Here's how the part is built. I have some questions about the finished solid (model axes, mm). Face numbers are marked on the shaded views. Round coordinates to 2 decimals unless told otherwise and drop trailing zeros. Order: outer loops, then holes, each group sorted by start corner. A loop starts at its lowest first (then second) coordinate and runs counter-clockwise, first axis right, second up. Notation, with made-up numbers: M -8.5,18.25 L 32.5,18.25 A18 ccw 32.5,50.25 Z; hole C 25.5,10.25 d11. An arc over 180 degrees is marked long. Use one line per item in the form item = value. Start each with the question number.
Autodesk Inventor part; units mm, degrees
ref_plane "YZ Plane" through (0, 0, 0) normal (1, 0, 0) x (0, 1, 0)
ref_plane "XZ Plane" through (0, 0, 0) normal (0, 1, 0) x (-1, 0, 0)
ref_plane "XY Plane" through (0, 0, 0) normal (0, 0, 1) x (1, 0, 0)
sketch "Sketch1" plane through (0, 0, 0) normal (0, 1, 0) x (-1, 0, 0)
  line L0 (37.592, 37.592) -> (-37.592, 37.592)
  line L1 (-37.592, 37.592) -> (-37.592, -37.592)
  line L2 (-37.592, -37.592) -> (37.592, -37.592)
  line L3 (37.592, -37.592) -> (37.592, 37.592)
  line L4 (48.9249, 50.7063) -> (48.9249, -4.5387)
  line L5 (37.592, 0) -> (0, 0)
  line L6 (0, 0) -> (0, -37.592)
  point P0 (0, 0)
  dimension "d0" = 75.184
  dimension "d1" = 75.184
extrude "Extrusion1" add sketch "Sketch1" along normal blind 7.366
sketch "Sketch6" plane through (0, 7.366, 0) normal (0, 1, 0) x (1, 0, 0)
  line L0 (0, 0) -> (0, 25.4)
  line L1 (0, 25.4) -> (-25.4, 25.4)
  line L2 (-25.4, 25.4) -> (-25.4, -25.4)
  line L3 (-25.4, -25.4) -> (25.4, -25.4)
  line L4 (25.4, -25.4) -> (25.4, 25.4)
  circle A0 centre (25.4, 25.4) radius 3.302
  circle A1 centre (25.4, 25.4) radius 4.826
  circle A2 centre (25.4, -25.4) radius 3.302
  circle A3 centre (25.4, -25.4) radius 4.826
  circle A4 centre (-25.4, -25.4) radius 3.302
  circle A5 centre (-25.4, -25.4) radius 4.826
  circle A6 centre (-25.4, 25.4) radius 3.302
  circle A7 centre (-25.4, 25.4) radius 4.826
  dimension "d35" = 25.4
  dimension "d36" = 25.4
  dimension "d37" = 50.8
  dimension "d38" = 50.8
  dimension "d39" = 6.604
  dimension "d40" = 9.652
  dimension "d41" = 6.604
  dimension "d42" = 9.652
  dimension "d43" = 6.604
  dimension "d44" = 9.652
  dimension "d45" = 6.604
  dimension "d46" = 9.652
sketch "Sketch2" plane through (0, 7.366, 0) normal (0, 1, 0) x (1, 0, 0)
  line L0 (0, 0) -> (0, 12.7)
  line L1 (0, 12.7) -> (-12.7, 12.7)
  line L2 (-12.7, 12.7) -> (12.7, 12.7)
  line L3 (12.7, 12.7) -> (12.7, -12.7)
  line L4 (12.7, -12.7) -> (-12.7, -12.7)
  circle A0 centre (-12.7, -12.7) radius 3.302
  circle A1 centre (-12.7, -12.7) radius 4.826
  circle A2 centre (-12.7, 12.7) radius 3.302
  circle A3 centre (-12.7, 12.7) radius 4.826
  circle A4 centre (12.7, -12.7) radius 3.302
  circle A5 centre (12.7, -12.7) radius 4.826
  circle A6 centre (12.7, 12.7) radius 3.302
  circle A7 centre (12.7, 12.7) radius 4.826
  dimension "d4" = 12.7
  dimension "d5" = 12.7
  dimension "d6" = 25.4
  dimension "d7" = 25.4
  dimension "d8" = 25.4
  dimension "d9" = 6.604
  dimension "d10" = 9.652
  dimension "d11" = 6.604
  dimension "d12" = 9.652
  dimension "d13" = 6.604
  dimension "d14" = 9.652
  dimension "d15" = 6.604
  dimension "d16" = 9.652
sketch "Sketch3" plane through (-37.592, 0, 37.592) normal (0, 0, 1) x (1, 0, 0)
  point P0 (37.592, 0)
sketch "Sketch4" plane through (0, 0, 0) normal (0, -1, 0) x (1, 0, 0)
  line L0 (-37.592, 37.592) -> (38.608, 37.592)
  line L1 (38.608, 37.592) -> (38.608, 41.402)
  line L2 (38.608, 41.402) -> (-37.592, 41.402)
  line L3 (-37.592, 41.402) -> (-37.592, 37.592)
  line L4 (37.592, -37.592) -> (-37.592, -37.592)
  line L5 (-37.592, -37.592) -> (38.608, -37.592)
  line L6 (38.608, -37.592) -> (38.608, -41.402)
  line L7 (38.608, -41.402) -> (-37.592, -41.402)
  line L8 (-37.592, -41.402) -> (-37.592, -37.592)
  line L9 (37.592, 37.592) -> (37.592, 41.402)
  line L10 (37.592, -37.592) -> (37.592, -41.402)
  point P0 (0, 0)
  point P1 (38.1, -38.1)
  dimension "d21" = 3.81
  dimension "d22" = 3.81
extrude "Extrusion4" add sketch "Sketch4" against normal blind 16.002 contours L3 L2 L9 L0 | L10 L7 L8 L4
sketch "Sketch5" plane through (-37.592, 0, 41.402) normal (0, 0, 1) x (1, 0, 0)
  line L0 (0, 7.366) -> (75.184, 7.366)
  line L1 (75.184, 7.366) -> (70.612, 7.366)
  line L2 (70.612, 7.366) -> (70.612, 11.938)
  line L3 (0, 7.366) -> (4.572, 7.366)
  line L4 (4.572, 7.366) -> (4.572, 11.938)
  circle A0 centre (4.572, 11.938) radius 2.286
  circle A1 centre (70.612, 11.938) radius 2.286
  point P0 (37.592, 0)
  dimension "d25" = 4.572
  dimension "d26" = 4.572
  dimension "d27" = 4.572
  dimension "d51" = 4.572
  dimension "d52" = 4.572
extrude "Extrusion5" cut sketch "Sketch6" against normal blind 25.4 contours A0 | A6 L2 L1 | L1 L2 A6 | A4 L3 L2 | L2 L3 A4 | A2 L4 L3 | L3 L4 A2
extrude "Extrusion6" cut sketch "Sketch6" against normal blind 6.604 contours A7 L2 A6 L1 | L1 A6 L2 A7 | A0 | A1 | A3 L4 A2 L3 | L3 A2 L4 A3 | A5 L3 A4 L2 | L2 A4 L3 A5 | A6 L2 L1 | L1 L2 A6 | A4 L3 L2 | L2 L3 A4 | A2 L4 L3 | L3 L4 A2
extrude "Extrusion7" cut sketch "Sketch5" against normal blind 127
properties part number "Voicecoil_to_PY004_Coupler"
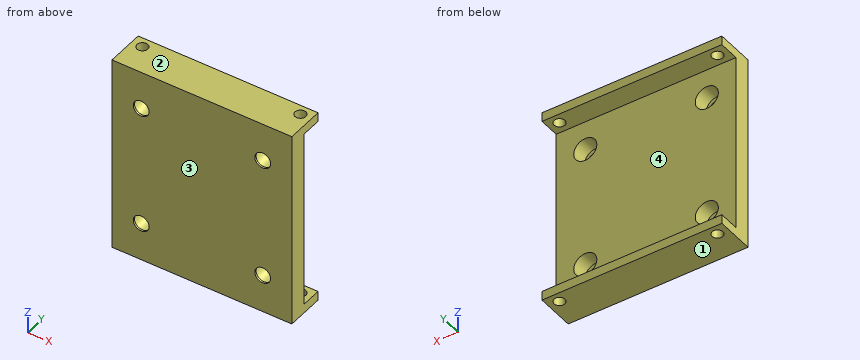
1) Will these pins go through, and if not, where does the flat tip stop? pin 1 Ø3 at (x, z) = (27, 25) entering from +Y; pin 2 Ø8 at (x, z) = (23.5, 3) entering from +Y; pin 3 Ø8 at (y, z) = (8.5, 13) entering from +X.
2) If I drill on line 1 (Z direction, x = 25.4, y = 0.4); line 2 (X direction, y = 0.4, z = -25.4); line 3 (Y direction, x = 33.02, z = 39.4), over which ranges is the centre line in solid material (lowest first)?
3) If we mould it in two halves opening along Z, with no side actions, what happens to the marked faces 1, 2, 3 and 4? For each: +Z half, -Z half, draft (parallel to the pull), parting line (faces both ways), or undercut.
4) If we section it at A-A on z = -25.4: Write out the boundary of the cut face in (x, y).
5) If we section it at C-C on y = 3: Write out the boundary of the cut face in (x, z).
6) If we section it at B-B on x = 33.02: Write out the boundary of the cut face in (y, z), then the cut area to 3 significant figures.
7) If we section it at D-D on x = 25.4: Write out the boundary of the cut face in (y, z), then the cut area to 3 significant figures.
Completed:
q1.pin_1 = through
q1.pin_2 = 7.37
q1.pin_3 = 37.59
q2.line_1 = -41.4 to -28.7, -22.1 to 22.1, 28.7 to 41.4
q2.line_2 = -37.59 to -28.7, -22.1 to 22.1, 28.7 to 37.59
q2.line_3 = 0 to 9.65, 14.22 to 16
q3.face_1 = -Z half
q3.face_2 = +Z half
q3.face_3 = draft
q3.face_4 = undercut
q4.outline = M -37.59,0 L -28.7,0 L -28.7,0.76 L -30.23,0.76 L -30.23,7.37 L -37.59,7.37 Z; M -22.1,0 L 22.1,0 L 22.1,0.76 L 20.57,0.76 L 20.57,7.37 L -20.57,7.37 L -20.57,0.76 L -22.1,0.76 Z; M 28.7,0 L 37.59,0 L 37.59,7.37 L 30.23,7.37 L 30.23,0.76 L 28.7,0.76 Z
q5.outline = M -37.59,-41.4 L 37.59,-41.4 L 37.59,41.4 L -37.59,41.4 Z; hole C -25.4,-25.4 d9.65; hole C -25.4,25.4 d9.65; hole C 25.4,-25.4 d9.65; hole C 25.4,25.4 d9.65
q6.outline = M 0,-41.4 L 9.65,-41.4 L 9.65,-37.59 L 7.37,-37.59 L 7.37,37.59 L 9.65,37.59 L 9.65,41.4 L 0,41.4 Z; M 14.22,-41.4 L 16,-41.4 L 16,-37.59 L 14.22,-37.59 Z; M 14.22,37.59 L 16,37.59 L 16,41.4 L 14.22,41.4 Z
q6.area = 641 mm²
q7.outline = M 0,-41.4 L 16,-41.4 L 16,-37.59 L 7.37,-37.59 L 7.37,-30.23 L 0.76,-30.23 L 0.76,-28.7 L 0,-28.7 Z; M 0,-22.1 L 0.76,-22.1 L 0.76,-20.57 L 7.37,-20.57 L 7.37,20.57 L 0.76,20.57 L 0.76,22.1 L 0,22.1 Z; M 0,28.7 L 0.76,28.7 L 0.76,30.23 L 7.37,30.23 L 7.37,37.59 L 16,37.59 L 16,41.4 L 0,41.4 Z
q7.area = 538 mm²
